Work out the finished part from the listing and answer in its coordinate system (mm). Coordinates: 2 decimals unless noted, no trailing zeros. Write each question's results on one line, items separated by ' | '.
```python
from build123d import *

# Parameters (mm, degrees)
SKETCH1_W                      = 304.8
SKETCH1_H                      = 63.5
BOSS_EXTRUDE1_DEPTH            = 9.525
F_5_16_18_TAPPED_HOLE1_D       = 6.5278
F_5_16_0_3125_DIAMETER_HOLE1_D = 7.9375
F_10_32_TAPPED_HOLE1_D         = 4.0386
F_10_32_TAPPED_HOLE1_DEPTH     = 11.938
F_10_32_TAPPED_HOLE1_TIP       = 1.213317848


with BuildPart() as part:
    # Sketch1 → Boss-Extrude1 (new body)
    with BuildSketch(Plane.XY):
        Rectangle(SKETCH1_W, SKETCH1_H)
    extrude(amount=BOSS_EXTRUDE1_DEPTH)

    # 5/16-18 Tapped Hole1 (through all)
    with Locations(Plane(origin=(-41.275, 23.114, 9.525), x_dir=(1, 0, 0), z_dir=(0, 0, 1))):
        with Locations((0, 0), (82.55, 0), (82.55, -38.1), (0, -38.1)):
            Hole(F_5_16_18_TAPPED_HOLE1_D / 2)

    # 5/16 (0.3125) Diameter Hole1 (through all)
    with Locations(Plane(origin=(-117.475, 22.225, 9.525), x_dir=(1, 0, 0), z_dir=(0, 0, 1))):
        with Locations((0, 0), (0, -44.323), (234.823, -44.323), (234.823, 0)):
            Hole(F_5_16_0_3125_DIAMETER_HOLE1_D / 2)

    # #10-32 Tapped Hole1
    with Locations(Plane(origin=(-139.7, 31.75, 4.445), x_dir=(0, 0, 1), z_dir=(0, 1, 0))):
        with Locations((0, 0), (0, 279.4)):
            Hole(F_10_32_TAPPED_HOLE1_D / 2, depth=F_10_32_TAPPED_HOLE1_DEPTH)
            with Locations((0, 0, -(F_10_32_TAPPED_HOLE1_DEPTH + F_10_32_TAPPED_HOLE1_TIP / 2))):  # 118° drill point
                Cone(0, F_10_32_TAPPED_HOLE1_D / 2, F_10_32_TAPPED_HOLE1_TIP, mode=Mode.SUBTRACT)


solid = part.part
```
1) For a pull along Y with two mould halves and no side action, classify faces 1 (the face through (-2, -31.75, 5)), 2 (the face through (-38.685, 21.128, 4.696)), 3 (the face through (-2, 0, 0)), 4 (the face through (121.313, -21.924, 4.696)) as released by +Y, released by -Y, zero draft, split by the parting line, or undercut.
Check result:
face 1: released by -Y | face 2: undercut | face 3: zero draft | face 4: undercut
2) Straight lines are drawn through the part: probe 1 along X at (y, z) = (-25, 3.75); probe 2 along X at (y, z) = (23, 2.25); probe 3 along X at (y, z) = (-12, 4.5). For each, find the intervals that lie inside material, in ascending order. Write a range as [from, to].
Check result:
probe 1: [-152.4, -120.18], [-114.77, 114.64], [120.06, 152.4] | probe 2: [-152.4, -121.37], [-113.58, -44.54], [-38.01, 38.01], [44.54, 113.46], [121.24, 152.4] | probe 3: [-152.4, -42.59], [-39.96, 39.96], [42.59, 152.4]
3) Given pin 1 Ø6 at (x, y) = (-41.275, -14.986) entering from +Z; pin 2 Ø3 at (x, z) = (139.7, 4.445) entering from +Y, each flat-ended and moving along its own axis, determine where each tip first touches the part or whether it passes through.
Check result:
pin 1: through | pin 2: y = 19.5
